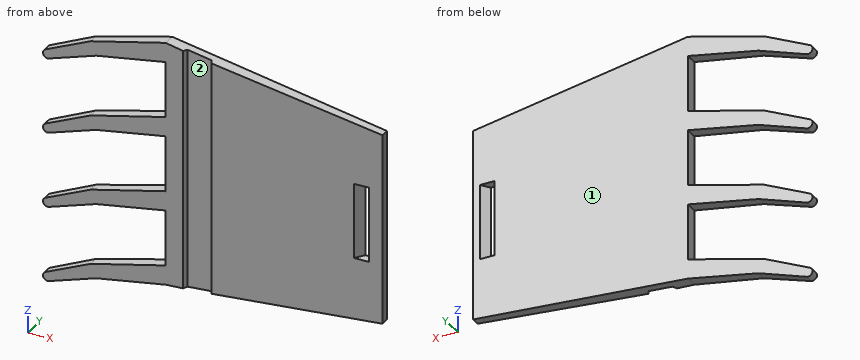
```python
from build123d import *

# Parameters (mm, degrees)
BOSS_EXTRUDE1_START = 28
BOSS_EXTRUDE1_DEPTH = 99.579374
SKETCH1_OUTSIDE_W   = 155.246
SKETCH1_OUTSIDE_H   = 133.053
CUT_EXTRUDE1_DEPTH  = 96.54042058
CUT_EXTRUDE2_START  = -32.303625
CUT_EXTRUDE2_DEPTH  = 27


with BuildPart() as part:
    # Sketch2 → Boss-Extrude1 (new body)
    with BuildSketch(Plane.XY.offset(BOSS_EXTRUDE1_START)):
        Polygon((-58.652152565, -2.957030561), (-7.219837935, -4.5), (-6.431436891, -3), (2.141659611, -3), (2.930060654, -4.5), (63.119847768, -3), (63.119847768, 0), (-58.652152565, 0), align=None)
    extrude(amount=-BOSS_EXTRUDE1_DEPTH)

    # Sketch1 outside → Cut-Extrude1 (cut, through all)
    with BuildSketch(Plane(origin=(0, 0, 0), x_dir=(1, 0, 0), z_dir=(0, 1, 0))):
        with Locations((2.234, 21.7895)):
            Rectangle(SKETCH1_OUTSIDE_W, SKETCH1_OUTSIDE_H)
        with BuildLine():
            Line((-40.711846446, -20.63757447), (-13.556580584, -28))
            Line((-13.556580584, -28), (63.119847768, -15.031886942))
            Line((63.119847768, -15.031886942), (63.119847768, 53.565574166))
            Line((63.119847768, 53.565574166), (-13.556580584, 60))
            Line((-13.556580584, 60), (-38.779919931, 65.060888634))
            Line((-38.779919931, 65.060888634), (-55.906958074, 71.115272488))
            ThreePointArc((-55.906958074, 71.115272488), (-57.932881972, 70.210638871), (-57.133307602, 68.140998698))
            Line((-57.133307602, 68.140998698), (-40.711846446, 60.36242553))
            Line((-40.711846446, 60.36242553), (-13.556580584, 53))
            Line((-13.556580584, 53), (-13.556580584, 33))
            Line((-13.556580584, 33), (-38.779919931, 38.060888634))
            Line((-38.779919931, 38.060888634), (-55.906958074, 44.115272488))
            ThreePointArc((-55.906958074, 44.115272488), (-57.932881972, 43.210638871), (-57.133307602, 41.140998698))
            Line((-57.133307602, 41.140998698), (-40.711846446, 33.36242553))
            Line((-40.711846446, 33.36242553), (-13.556580584, 26))
            Line((-13.556580584, 26), (-13.556580584, 6))
            Line((-13.556580584, 6), (-38.779919931, 11.060888634))
            Line((-38.779919931, 11.060888634), (-55.906958074, 17.115272488))
            ThreePointArc((-55.906958074, 17.115272488), (-57.932881972, 16.210638871), (-57.133307602, 14.140998698))
            Line((-57.133307602, 14.140998698), (-40.711846446, 6.36242553))
            Line((-40.711846446, 6.36242553), (-13.556580584, -1))
            Line((-13.556580584, -1), (-13.556580584, -21))
            Line((-13.556580584, -21), (-38.779919931, -15.939111366))
            Line((-38.779919931, -15.939111366), (-55.906958074, -9.884727512))
            ThreePointArc((-55.906958074, -9.884727512), (-57.932881972, -10.789361129), (-57.133307602, -12.859001302))
            Line((-57.133307602, -12.859001302), (-40.711846446, -20.63757447))
        make_face(mode=Mode.SUBTRACT)
    extrude(amount=-CUT_EXTRUDE1_DEPTH, mode=Mode.SUBTRACT)

    # Sketch3 → Cut-Extrude2 (cut)
    with BuildSketch(Plane.XY.offset(CUT_EXTRUDE2_START)):
        Polygon((60.602138865, 0), (55.427246155, 0), (53.07800672, -3.250254442), (58.455951346, -3.116229762), align=None)
    extrude(amount=CUT_EXTRUDE2_DEPTH, mode=Mode.SUBTRACT)


solid = part.part
```
Input: part model. Units: mm. Frame: model coordinates. Face numbers are marked on the shaded views. A direction names the side the tool comes from. Round coordinates to 2 decimals unless told otherwise and drop trailing zeros. Write each loop counter-clockwise with the first axis right and the second up, starting at its lowest first coordinate (ties: lowest second). Pieces come first, ordered by that corner, then holes. Notation, with made-up numbers: (18.5, -30.75) -> (67.5, -30.75) arc R17 cw to (67.5, -26.75) -> close; hole circle Ø3 at (-5, 9). An arc over 180 degrees is marked (long way). Answer as CSV lines item,"result".
1. Section A-A (x = -43). Return the cut outline in (y, z).
Geometry says:
outline,"(-3.43, -66.55) -> (0, -66.55) -> (0, -61.45) -> (-3.43, -61.45) -> close; (-3.43, -39.55) -> (0, -39.55) -> (0, -34.45) -> (-3.43, -34.45) -> close; (-3.43, -12.55) -> (0, -12.55) -> (0, -7.45) -> (-3.43, -7.45) -> close; (-3.43, 14.45) -> (0, 14.45) -> (0, 19.55) -> (-3.43, 19.55) -> close"
2. Contact query for flat-ended pins moving along their axis: P1, Ø1.3, axis at y = -3, z = -15, coming from the -X side; P2, Ø2.5, axis at x = 58, y = -2.5, coming from the -Z side; P3, Ø8, axis at x = -42.5, z = -40.5, coming from the -Y side; P4, Ø1.6, axis at x = 57.5, y = -1, coming from the +Z side. Output: stop coordinate, or through.
Geometry says:
P1,"stops at x = -58.05"
P2,"stops at z = -54.1"
P3,"stops at y = -3.54"
P4,"stops at z = 16.12"
3. Section D-D (x = -29). Return the cut outline in (y, z).
Geometry says:
outline,"(-3.85, -63.1) -> (0, -63.1) -> (0, -57.19) -> (-3.85, -57.19) -> close; (-3.85, -36.1) -> (0, -36.1) -> (0, -30.19) -> (-3.85, -30.19) -> close; (-3.85, -9.1) -> (0, -9.1) -> (0, -3.19) -> (-3.85, -3.19) -> close; (-3.85, 17.9) -> (0, 17.9) -> (0, 23.81) -> (-3.85, 23.81) -> close"
4. Ray query, L1, parallel to Z at x = -20.5, y = -2.2; L2, parallel to Z at x = -36.5, y = -1; L3, parallel to Y at x = 40.5, z = -48.5. Return the intervals inside material, ascending. Write a range as [from, to].
Geometry says:
L1,"z = [-61.39, -54.88], [-34.39, -27.88], [-7.39, -0.88], [19.61, 26.12]"
L2,"z = [-64.6, -59.22], [-37.6, -32.22], [-10.6, -5.22], [16.4, 21.78]"
L3,"y = [-3.56, 0]"
5. Section B-B (z = -39.5). Return the cut outline in (x, y).
Geometry says:
outline,"(-53.67, -3.11) -> (-42.85, -3.43) -> (-42.85, 0) -> (-53.67, 0) -> close; (-13.56, -4.31) -> (-7.22, -4.5) -> (-6.43, -3) -> (2.14, -3) -> (2.93, -4.5) -> (63.12, -3) -> (63.12, 0) -> (-13.56, 0) -> close"
6. Reachability of the marked faces 1 and 2 from +Z, -Z, +X, -X, +Y, -Y: full face, straight path, thin tool, end or side. Return the list, or none.
Geometry says:
face 1,"+Z, -Z, +X, -X, +Y"
face 2,"+Z, -Z, -Y"
